Source: CAD feature listing. Evaluate the final solid. Frame: model axes, mm. A direction names the side the tool comes from. Give positions to 0.01 mm unless a question says otherwise; leave off trailing zeros. Order: outer loops, then holes, each group sorted by start corner. A loop starts at its lowest first (then second) coordinate and runs counter-clockwise, first axis right, second up. Notation, with made-up numbers: (21.25, 87.5) - (77.25, 87.5) arc R10 ccw to (77.25, 105.5) - close; hole circle Ø6 at (49, 81). An arc over 180 degrees is marked (long way). Answer as CSV lines item,"result".
```python
from build123d import *

# Parameters (mm, degrees)
F0_W     = 33
F0_H     = 1
F0_H_2   = 15
F0_R     = 1.5
F0_W_2   = 9
F0_H_3   = 13
F1_DEPTH = 18
F3_DEPTH = 17.001
F4_R     = 1.5
F5_DEPTH = 17.001
F6_R     = 3
F7_DEPTH = 4.5
F8_DEPTH = 1
F9_DEPTH = 1


with BuildPart() as f1:
    # F0 (on Top) → F1 (new body)
    with BuildSketch(Plane.XY):
        with Locations((16.5, 0.5)):
            Rectangle(F0_W, F0_H)
        with Locations((16.5, 8.5)):
            Rectangle(F0_W, F0_H_2)
        with Locations((7.5, 8.5)):
            Circle(F0_R, mode=Mode.SUBTRACT)
        with Locations((27.5, 8.5)):
            Rectangle(F0_W_2, F0_H_3, mode=Mode.SUBTRACT)
        with Locations((16.5, 16.5)):
            Rectangle(F0_W, F0_H)
    extrude(amount=-F1_DEPTH)

    # F2 (on face) → F3 (cut, through all)
    with BuildSketch(Plane.XZ):
        Polygon((5, -18), (0, 0), (0, -18), align=None)
    extrude(amount=-F3_DEPTH, mode=Mode.SUBTRACT)

    # F4 (on face) → F5 (cut, through all)
    with BuildSketch(Plane.XZ):
        with Locations((12, -9)):
            Circle(F4_R)
        with BuildLine():
            ThreePointArc((16.9193976722, -15.5707030324), (20.2081866768, -9.0168308246), (16.9463025453, -2.4495265112))
            ThreePointArc((16.9463025453, -2.4495265112), (14.8453357329, -2.7426791223), (15.138488344, -4.8436459346))
            ThreePointArc((15.138488344, -4.8436459346), (17.2081929835, -9.0106793603), (15.1214168791, -13.1691899537))
            ThreePointArc((15.1214168791, -13.1691899537), (14.8196507362, -15.2689368896), (16.9193976722, -15.5707030324))
        make_face()
    extrude(amount=-F5_DEPTH, mode=Mode.SUBTRACT)

    # F6 (on face) → F7 (cut)
    with BuildSketch(Plane(origin=(0, 0, -18), x_dir=(1, 0, 0), z_dir=(0, 0, -1))):
        with Locations((7.5, -8.5)):
            Circle(F6_R)
    extrude(amount=-F7_DEPTH, mode=Mode.SUBTRACT)

    # F0 (on Top) → F8 (join)
    with BuildSketch(Plane.XY):
        with Locations((16.5, 16.5)):
            Rectangle(F0_W, F0_H)
        with Locations((16.5, 0.5)):
            Rectangle(F0_W, F0_H)
    extrude(amount=F8_DEPTH)

    # F9 (add): faces of the model
    f9_faces = [f1.faces().sort_by_distance(p)[0] for p in [
        (16.5, 16.5, 1),
        (16.5, 0.5, 1),
    ]]
    extrude(f9_faces, amount=F9_DEPTH)


solid = f1.part
```
(1) Cut plane A-A (z = -9). Return loops of the section in (x, y).
Completed:
outline,"(2.5, 0) - (10.5, 0) - (10.5, 17) - (2.5, 17) - close; (13.5, 0) - (17.21, 0) - (17.21, 17) - (13.5, 17) - close; (20.21, 0) - (33, 0) - (33, 17) - (20.21, 17) - close; hole circle Ø3 at (7.5, 8.5); hole (23, 2) - (32, 2) - (32, 15) - (23, 15) - close"
(2) Cut plane B-B (x = 12). Return loops of the section in (y, z), then the cut area to 3 significant figures.
Completed:
outline,"(0, -18) - (17, -18) - (17, -10.5) - (0, -10.5) - close; (0, -7.5) - (17, -7.5) - (17, 2) - (16, 2) - (16, 0) - (1, 0) - (1, 2) - (0, 2) - close"
area,"259 mm²"
(3) Cut plane C-C (y = 8). Return loops of the section in (x, z), then the cut area to 3 significant figures.
Completed:
outline,"(0, 0) - (4.54, -16.35) - (4.54, -13.5) - (6.09, -13.5) - (6.09, 0) - close; (8.91, -13.5) - (10.46, -13.5) - (10.46, -18) - (23, -18) - (23, 0) - (8.91, 0) - close; (32, -18) - (33, -18) - (33, 0) - (32, 0) - close; hole circle Ø3 at (12, -9); hole (15.12, -13.17) arc R1.5 ccw to (16.92, -15.57) arc R8.21 ccw to (16.95, -2.45) arc R1.5 ccw to (15.14, -4.84) arc R5.21 cw to start"
area,"271 mm²"
(4) Contact query for flat-ended pins moving along their axis: pin 1 (1 mm diameter, centred on y = 9, z = -9, fed in from -X); pin 2 (5.5 mm diameter, centred on x = 7.5, y = 8.5, fed in from +Z); pin 3 (2 mm diameter, centred on x = 8.5, y = 8, fed in from -Z). Output: stop coordinate, or through.
Completed:
pin 1,"x = 2.36"
pin 2,"z = 0"
pin 3,"z = -13.5"
(5) Access query for faces 5 (the cylindrical face through (10.36, 7.6, -15.78)), 6 (the flat face through (16.3, 16.5, 2)), 7 (the flat face through (16, 1, 1)), 8 (the flat face through (23, 8, -9)). Directions: +Z, -Z, +X, -X, +Y, -Y. A direction counts if a zero-diameter tool reaches every point of the face in a straight line with its end or side. Return the directions, or none.
Completed:
face 5,"-Z"
face 6,"+Z, +X, -X, +Y, -Y"
face 7,"+Z, +X, -X"
face 8,"+Z, -Z"
(6) Cut plane D-D (z = -5.25). Return loops of the section in (x, y), then the cut area to 3 significant figures.
Completed:
outline,"(1.46, 0) - (15.61, 0) - (15.61, 17) - (1.46, 17) - close; (19.3, 0) - (33, 0) - (33, 17) - (19.3, 17) - close; hole circle Ø3 at (7.5, 8.5); hole (23, 2) - (32, 2) - (32, 15) - (23, 15) - close"
area,"349 mm²"
(7) Ray query, line 1 (Y direction, x = 7.5, z = -9.5); line 2 (Y direction, x = 7.5, z = -16.75); line 3 (X direction, y = 15.75, z = -8). Return the intervals inside material, ascending. Write a range as from..to.
Completed:
line 1,"0..7, 10..17"
line 2,"0..5.5, 11.5..17"
line 3,"2.22..10.88, 13.12..17.11, 20.15..33"
(8) Mould query, pull axis Y, two halves, no side actions, for faces 1 (the flat face through (27, 15, -9)), 2 (the flat face through (16, 16, 1)), 3 (the cylindrical face through (14.866, 8.381, -2.717)), 4 (the flat face through (16, 0, -8)). Classes: released by +Y, released by -Y, zero draft, split by the parting line, or undercut.
Completed:
face 1,"undercut"
face 2,"undercut"
face 3,"zero draft"
face 4,"released by -Y"
